```python
from build123d import *

# Parameters (mm, degrees)
SKETCH3_R           = 17.5
SKETCH3_R_2         = 7.5
BOSS_EXTRUDE1_DEPTH = 15
SKETCH4_R           = 15
SKETCH4_R_2         = 10.5
CUT_EXTRUDE1_DEPTH  = 1
CUT_EXTRUDE2_START  = -1
SKETCH5_R           = 15
SKETCH5_R_2         = 10.5
CUT_EXTRUDE2_DEPTH  = 1


with BuildPart() as part:
    # Sketch3 → Boss-Extrude1 (new body)
    with BuildSketch(Plane.XY):
        Circle(SKETCH3_R)
        Circle(SKETCH3_R_2, mode=Mode.SUBTRACT)
    extrude(amount=BOSS_EXTRUDE1_DEPTH)

    # Sketch4 → Cut-Extrude1 (cut)
    with BuildSketch(Plane.XY.offset(15)):
        Circle(SKETCH4_R)
        Circle(SKETCH4_R_2, mode=Mode.SUBTRACT)
    extrude(amount=-CUT_EXTRUDE1_DEPTH, mode=Mode.SUBTRACT)

    # Sketch5 → Cut-Extrude2 (cut)
    with BuildSketch(Plane(origin=(0, 0, 0), x_dir=(-1, 0, 0), z_dir=(0, 0, -1)).offset(CUT_EXTRUDE2_START)):
        with Locations(Location((0, 0, 0), (0, 0, 180))):
            Circle(SKETCH5_R)
        with Locations(Location((0, 0, 0), (0, 0, 180))):
            Circle(SKETCH5_R_2, mode=Mode.SUBTRACT)
    extrude(amount=CUT_EXTRUDE2_DEPTH, mode=Mode.SUBTRACT)


solid = part.part
```
Verification items for the finished model (mm, model axes). A direction names the side the tool comes from. Coordinates: 2 decimals unless noted, no trailing zeros. Loops run counter-clockwise (first coordinate to the right, second up) from the corner with the lowest first, then second, coordinate; pieces in that order, holes last. Notation, with made-up numbers: (45, 33.5) -> (62, 33.5) arc R21 ccw to (62, 63.5) -> close; hole circle Ø1 at (44.5, 43). An arc over 180 degrees is marked (long way). Put each result on its own line as item: value.
1. Section check A-A, the plane y = 0. Record the boundary of the cut face in (x, z).
Result set:
outline: (-17.5, 0) -> (-15, 0) -> (-15, 1) -> (-10.5, 1) -> (-10.5, 0) -> (-7.5, 0) -> (-7.5, 15) -> (-10.5, 15) -> (-10.5, 14) -> (-15, 14) -> (-15, 15) -> (-17.5, 15) -> close; (7.5, 0) -> (10.5, 0) -> (10.5, 1) -> (15, 1) -> (15, 0) -> (17.5, 0) -> (17.5, 15) -> (15, 15) -> (15, 14) -> (10.5, 14) -> (10.5, 15) -> (7.5, 15) -> close
2. Tool access check on faces 1 (the face through (10, 3.2, 14.5)), 2 (the face through (5, -7, 0)), 3 (the face through (8.06, -12.65, 0.51)). Record the directions out of +Z, -Z, +X, -X, +Y, -Y that give a thin tool (end or side, any length) a straight path to the whole face; none if there is none.
Result set:
face 1: +Z
face 2: -Z, +X, -X, +Y, -Y
face 3: -Z
3. Thickness scan on line 1 (Y direction, x = 0, z = 0.45); line 2 (Y direction, x = 0, z = 6.75); line 3 (X direction, y = -6.5, z = 6.75). Record the ranges inside material, lowest first.
Result set:
line 1: y = -17.5 to -15, -10.5 to -7.5, 7.5 to 10.5, 15 to 17.5
line 2: y = -17.5 to -7.5, 7.5 to 17.5
line 3: x = -16.25 to -3.74, 3.74 to 16.25
4. Mould release check, pull along Y, two halves, no side actions. Record for faces 4 (the face through (-7.493, 0.33, 7.395)), 5 (the face through (13, 8, 15)), 6 (the face through (-13.887, -10.648, 7.395)): pulls with the +Y half, pulls with the -Y half, needs draft (parallel to the pull), parting line crosses it, or undercut.
Result set:
face 4: undercut
face 5: needs draft
face 6: parting line crosses it
5. Section check C-C, the plane z = 9.25. Record the boundary of the cut face in (x, y), then the cut area to 3 significant figures.
Result set:
outline: circle Ø35 at (0, 0); hole circle Ø15 at (0, 0)
area: 785 mm^2
6. Gauge pin test, flat ends, axial feed: P1, Ø4, axis at y = 9.5, z = 10, coming from the +X side; P2, Ø1, axis at x = 1.5, z = 9.5, coming from the -Y side; P3, Ø5, axis at y = -5.5, z = 12, coming from the +X side. Record the tip position at first contact, or that the pin passes through.
Result set:
P1: stops at x = 15.81
P2: stops at y = -17.47
P3: stops at x = 17.24
